```python
from build123d import *

# Parameters (mm, degrees)
F0_W     = 20
F0_H     = 20
F1_DEPTH = 20
F2_DEPTH = 20
F3_D     = 2
F3_DEPTH = 5
F3_TIP   = 0.600860619
F5_D     = 2
F5_DEPTH = 5
F5_TIP   = 0.600860619
F7_D     = 3


with BuildPart() as f1:
    # F0 (on Top) → F1 (new body)
    with BuildSketch(Plane.XY):
        with Locations((-7.549341768, 7.9021853259)):
            Rectangle(F0_W, F0_H)
    extrude(amount=F1_DEPTH)

    # F0 (on Top) → F2 (join)
    with BuildSketch(Plane.XY):
        with Locations((-7.549341768, 7.9021853259)):
            Rectangle(F0_W, F0_H)
    extrude(amount=F2_DEPTH)

    # F3
    with Locations(Plane(origin=(0, 0, 0), x_dir=(1, 0, 0), z_dir=(0, 0, -1))):
        with Locations((-12.8782894462, -7.9021853259), (-2.5164496619, -7.9021853259)):
            Hole(F3_D / 2, depth=F3_DEPTH)
            with Locations((0, 0, -(F3_DEPTH + F3_TIP / 2))):  # 118° drill point
                Cone(0, F3_D / 2, F3_TIP, mode=Mode.SUBTRACT)

    # F5
    with Locations(Plane.XY.offset(20)):
        with Locations((-12.8782894462, 7.9021853259), (-2.6713556144, 7.9021853259)):
            Hole(F5_D / 2, depth=F5_DEPTH)
            with Locations((0, 0, -(F5_DEPTH + F5_TIP / 2))):  # 118° drill point
                Cone(0, F5_D / 2, F5_TIP, mode=Mode.SUBTRACT)

    # F7 (through all)
    with Locations(Plane.XZ.offset(2.0978146741)):
        with Locations((-12.5512500335, 10.0038165309), (-2.3071385143, 10.0038165309)):
            Hole(F7_D / 2)


solid = f1.part
```
Could you check a few things on this model? Use its own coordinates, in mm. A direction names the side the tool comes from. Round coordinates to 2 decimals unless told otherwise and drop trailing zeros. Loops run counter-clockwise (first coordinate to the right, second up) from the corner with the lowest first, then second, coordinate; pieces in that order, holes last. Notation, with made-up numbers: M 23.5,50.25 L 59.5,50.25 A16 ccw 59.5,55.25 Z; hole C -3,-27 d9. An arc over 180 degrees is marked long. Write item = value, one per line.
1. Which directions (+Z, -Z, +X, -X, +Y, -Y) give clear straight access to the entire face, cutting with the end or side of a thin tool? Please do faces 1 (the face through (-2.98, 8.79, 2.54)), 2 (the face through (-8, 17.902, 10)), 3 (the face through (-1.88, 7.29, 17.46)).
Results below:
face_1 = -Z
face_2 = +Z, -Z, +X, -X, +Y
face_3 = +Z
2. Thinking about a two-plate mould opening in Z: for faces 4 (the face through (-8, -2.098, 10)), 5 (the face through (-13.016, 7.797, 14.503)), 6 (the face through (-8, 8, 0)), 7 (the face through (-2.999, 8.042, 8.673)), which applies, +Z half, -Z half, draft (parallel to the pull), parting line (faces both ways), or undercut?
Results below:
face_4 = draft
face_5 = +Z half
face_6 = -Z half
face_7 = undercut
3. Will these pins go through, and if not, where does the flat tip stop? P1, Ø1.6, axis at x = -2.67, y = 7.9, coming from the +Z side; P2, Ø8, axis at x = -4.5, y = 2.5, coming from the -Z side; P3, Ø1.8, axis at x = -12.88, y = 7.9, coming from the -Z side; P4, Ø2.5, axis at x = -12.55, z = 10, coming from the -Y side (1 decimal).
Results below:
P1 = 14.88
P2 = 0
P3 = 5.06
P4 = through
4. I want a section at D-D, the plane y = 7.5. Count the separate pieces of the cut face and the enclosed holes in it, and give its area (3 significant figures).
Results below:
separate_pieces = 1
enclosed_holes = 2
area = 348 mm²
5. I want a section at A-A, the plane z = 9.5. Write out the boundary of the cut face in (x, y), and give its area (3 significant figures).
Results below:
outline = M -17.55,-2.1 L -13.96,-2.1 L -13.96,17.9 L -17.55,17.9 Z; M -11.14,-2.1 L -3.72,-2.1 L -3.72,17.9 L -11.14,17.9 Z; M -0.89,-2.1 L 2.45,-2.1 L 2.45,17.9 L -0.89,17.9 Z
area = 287 mm²
6. I want a section at C-C, the plane z = 16. Write out the boundary of the cut face in (x, y), and give its area (3 significant figures).
Results below:
outline = M -17.55,-2.1 L 2.45,-2.1 L 2.45,17.9 L -17.55,17.9 Z; hole C -12.88,7.9 d2; hole C -2.67,7.9 d2
area = 394 mm²
7. I need wall thicknesses on probe 1 along X at (y, z) = (3.25, 9.25); probe 2 along X at (y, z) = (7, 3); probe 3 along Z at (x, y) = (-12.5, 11). Which ranges of each line are inside material? Lowest first, please.
Results below:
probe_1 = -17.55 to -13.85, -11.25 to -3.6, -1.01 to 2.45
probe_2 = -17.55 to -13.31, -12.45 to -2.95, -2.09 to 2.45
probe_3 = 0 to 8.5, 11.5 to 20
8. I want a section at B-B, the plane y = 14. Write out the boundary of the cut face in (x, z), and give its area (3 significant figures).
Results below:
outline = M -17.55,0 L 2.45,0 L 2.45,20 L -17.55,20 Z; hole C -12.55,10 d3; hole C -2.31,10 d3
area = 386 mm²
